CAD build for the part. Positions are in the model's coordinates, mm. Face numbers are marked on the shaded views. A direction names the side the tool comes from. Give positions to 0.01 mm unless a question says otherwise; leave off trailing zeros. Order: outer loops, then holes, each group sorted by start corner. A loop starts at its lowest first (then second) coordinate and runs counter-clockwise, first axis right, second up. Notation, with made-up numbers: M 10.5,13.25 L 28.5,13.25 A24 ccw 28.5,36.25 Z; hole C 17.25,35 d6. An arc over 180 degrees is marked long. Put each result on its own line as item: value. Start each with the question number.
1) Two-plate mould, pull along Y, no slides. Class the marked faces 1, 2, 3 and 4: released by +Y, released by -Y, zero draft, split by the parting line, or undercut.
2) Cut at D-D (y = 4.25). Write the cut outline in (x, z), and give its area (3 significant figures).
3) Drill centre lines: line 1 (X direction, y = 4.25, z = 1.85); line 2 (X direction, y = 0.5, z = 1.1). Where is each one in solid material? Low to high. Write a range as [from, to].
4) Cut at C-C (z = 2.55). Write the cut outline in (x, y).
5) Cut at B-B (y = 0). Write the cut outline in (x, z).
6) Tool access for the marked faces 5 and 6: list every direction of +Z, -Z, +X, -X, +Y, -Y with a clear straight run to the whole face (end or side of a thin tool).
7) Cut at A-A (x = 0). Write the cut outline in (y, z), and give its area (3 significant figures).
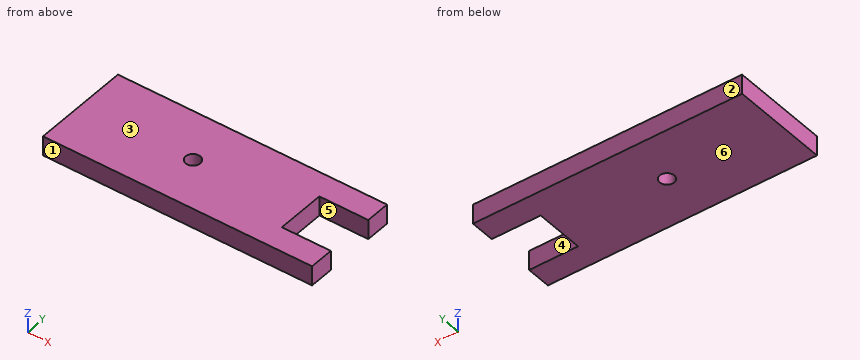
```python
from build123d import *

# Parameters (mm, degrees)
F0_R     = 1.5
F1_DEPTH = 4


with BuildPart() as f1:
    # F0 (on Top) → F1 (new body)
    with BuildSketch(Plane.XY):
        Polygon((-23, 10), (-23, 0), (-23, -10), (32, -10), (32, -5), (22, -5), (22, 0), (22, 5), (32, 5), (32, 10), align=None)
        Circle(F0_R, mode=Mode.SUBTRACT)
    extrude(amount=F1_DEPTH)


solid = f1.part
```
Solution:
1. face 1: released by -Y
1. face 2: released by +Y
1. face 3: zero draft
1. face 4: undercut
2. outline: M -23,0 L 22,0 L 22,4 L -23,4 Z
2. area: 180 mm²
3. line 1: [-23, 22]
3. line 2: [-23, -1.41], [1.41, 22]
4. outline: M -23,-10 L 32,-10 L 32,-5 L 22,-5 L 22,5 L 32,5 L 32,10 L -23,10 Z; hole C 0,0 d3
5. outline: M -23,0 L -1.5,0 L -1.5,4 L -23,4 Z; M 1.5,0 L 22,0 L 22,4 L 1.5,4 Z
6. face 5: +Z, -Z, +X
6. face 6: -Z, +X, -X, +Y, -Y
7. outline: M -10,0 L -1.5,0 L -1.5,4 L -10,4 Z; M 1.5,0 L 10,0 L 10,4 L 1.5,4 Z
7. area: 68.0 mm²
